Verification items for the finished model (mm, model axes). A direction names the side the tool comes from. Coordinates: 2 decimals unless noted, no trailing zeros. Loops run counter-clockwise (first coordinate to the right, second up) from the corner with the lowest first, then second, coordinate; pieces in that order, holes last. Notation, with made-up numbers: (3, 63) - (17, 63) arc R12 ccw to (17, 84) - close; hole circle Ø6 at (84, 20). An arc over 180 degrees is marked (long way). Answer as CSV lines item,"result". Start each with the question number.
1. Gauge pin test, flat ends, axial feed: P1, Ø1, axis at x = 5, z = -6.5, coming from the -Y side; P2, Ø4, axis at y = -4, z = -6.5, coming from the +X side; P3, Ø2, axis at y = -8.5, z = -4, coming from the +X side. Record the tip position at first contact, or that the pin passes through.
2. Material ranges on line 1 (X direction, y = 4.5, z = 11); line 2 (X direction, y = 6.25, z = 11); line 3 (Y direction, x = -2, z = -4), recorded low to high. Write a range as [from, to].
3. Set-up check for faces 1 (the flat face through (6.8, 10.7, -11.15)), 2 (the flat face through (10, -7, -18)), 3 (the flat face through (-8, -3, 17.645)): record each of +Z, -Z, +X, -X, +Y, -Y from which the full face is reachable in a straight line by a thin tool's end or side.
4. Cross-section at A-A (z = 16). Enter the section's corners in (x, y), plus the area to 3 significant figures.
5. Release check for a two-part mould opening along Z. For faces 4 (the flat face through (6.8, 10.7, 11.15)), 5 (the flat face through (-8, 3, -17.645)), 6 (the cylindrical face through (3.621, 11.497, -17.82)) record: pulls with the +Z half, pulls with the -Z half, needs draft (parallel to the pull), parting line crosses it, or undercut.
```python
from build123d import *

# Parameters (mm, degrees)
SKETCH3_W = 1.3
SKETCH3_H = 0.473161305


with BuildPart() as part:
    # Sketch2 → Body (revolve)
    with BuildSketch(Plane(origin=(0, 0, 0), x_dir=(0, 0, -1), z_dir=(1, 0, 0))):
        with BuildLine():
            Line((-17.645349183, 12.053677391), (-18, 12.053677391))
            Line((-18, 12.053677391), (-18, 12.526838695))
            ThreePointArc((-18, 12.526838695), (-17.861414262, 12.861414262), (-17.526838695, 13))
            Line((-17.526838695, 13), (17.526838695, 13))
            ThreePointArc((17.526838695, 13), (17.861414262, 12.861414262), (18, 12.526838695))
            Line((18, 12.526838695), (18, 12.053677391))
            Line((18, 12.053677391), (17.645349183, 12.053677391))
            Line((17.645349183, 12.053677391), (17.645349183, 8))
            Line((17.645349183, 8), (-17.645349183, 8))
            Line((-17.645349183, 8), (-17.645349183, 12.053677391))
        make_face()
    revolve(axis=Axis((0, 0, 18), (0, 0, -1)))

    # Sketch3 → Track (revolve, cut)
    with BuildSketch(Plane(origin=(0, 0, 0), x_dir=(0, 0, -1), z_dir=(1, 0, 0))):
        with Locations((11.8, 12.763419348)):
            Rectangle(SKETCH3_W, SKETCH3_H)
        with Locations((-11.8, 12.763419348)):
            Rectangle(SKETCH3_W, SKETCH3_H)
    revolve(axis=Axis((0, 0, 18), (0, 0, -1)), mode=Mode.SUBTRACT)


solid = part.part
```
Values follow:
1,P1,"stops at y = -12.2"
1,P2,"stops at x = 12.85"
1,P3,"stops at x = 10.62"
2,line 1,"x = [-12.2, -6.61], [6.61, 12.2]"
2,line 2,"x = [-11.4, -4.99], [4.99, 11.4]"
2,line 3,"y = [-12.85, -7.75], [7.75, 12.85]"
3,face 1,"none"
3,face 2,"-Z, +X, -X, +Y, -Y"
3,face 3,"+Z"
4,outline,"circle Ø26 at (0, 0); hole circle Ø16 at (0, 0)"
4,area,"330 mm²"
5,face 4,"undercut"
5,face 5,"pulls with the -Z half"
5,face 6,"needs draft"
